Check sheet for the drawn part. Datum: minimum x, y, z corner. Units: mm. Coordinates: 2 decimals unless noted, no trailing zeros. Order: outer loops, then holes, each group sorted by start corner. A loop starts at its lowest first (then second) coordinate and runs counter-clockwise, first axis right, second up.
Q1. Cross-section at A-A, the plane z = 116.5. Record the boundary of the cut face in (x, y).
Q2. Cross-section at B-B, the plane x = 57. Record the boundary of the cut face in (y, z).
Q3. Thickness scan on line 1 (Z direction, x = 200.5, y = 202.5); line 2 (X direction, y = 167, z = 160.5); line 3 (Y direction, x = 55.5, z = 30.5). Record the ranges inside material, lowest first.
Q4. Depth check by flat-ended pin: P1, Ø12, axis at x = 146, z = 227, coming from the +Y side; P2, Ø8, axis at y = 152, z = 131.5, coming from the +X side; P3, Ø1, axis at x = 118, z = 198, coming from the -Y side. Enter the tip coordinate at first touch or a pass-through.
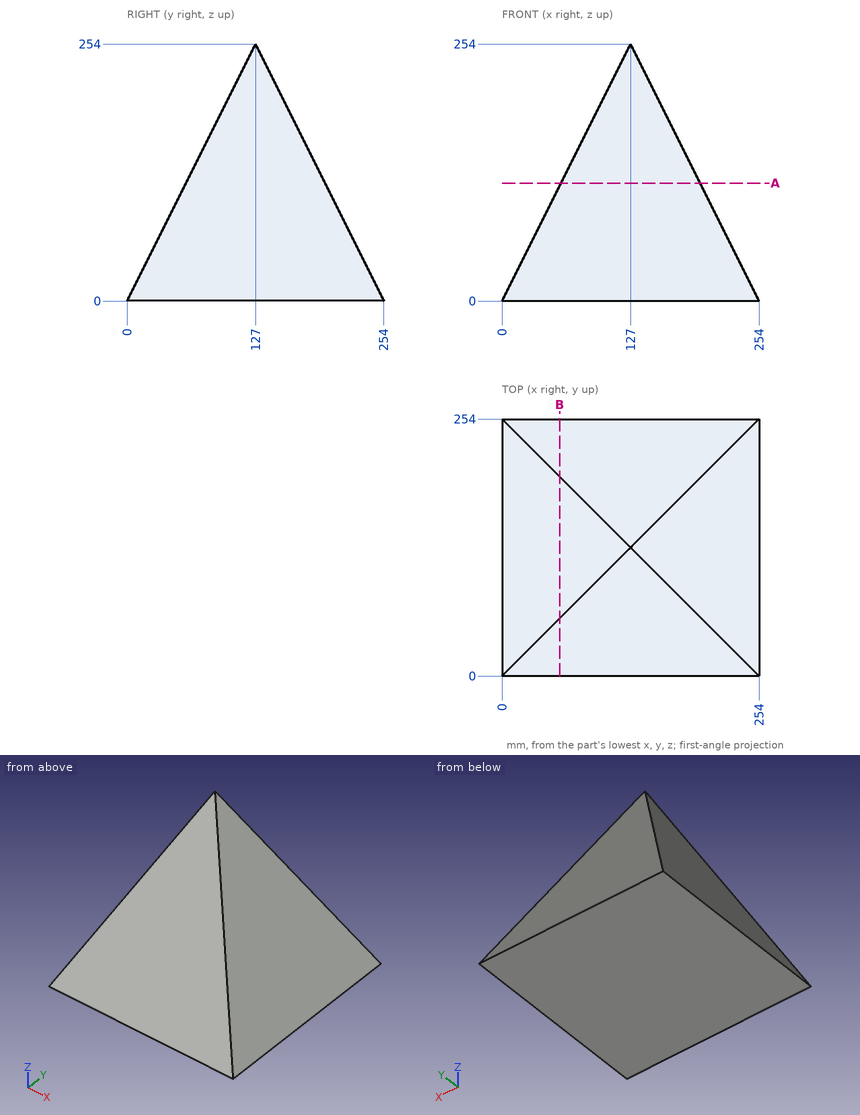
Check values:
1. outline: (58.25, 58.25) - (195.75, 58.25) - (195.75, 195.75) - (58.25, 195.75) - close
2. outline: (0, 0) - (254, 0) - (197, 114) - (57, 114) - close
3. line 1: z = 0 to 103
3. line 2: x = 80.25 to 173.75
3. line 3: y = 15.25 to 238.75
4. P1: stops at y = 143.14
4. P2: stops at x = 190.25
4. P3: stops at y = 98.75
